For this review, take the finished solid that the model builds, in its own axes (mm). Face numbers are marked on the shaded views. Give positions to 0.01 mm unless a question says otherwise; leave off trailing zeros. Loops run counter-clockwise (first coordinate to the right, second up) from the corner with the lowest first, then second, coordinate; pieces in that order, holes last. Notation, with made-up numbers: (84, 81) - (117, 81) arc R25 ccw to (117, 115) - close; hole circle Ø11 at (74, 39.25). An arc over 180 degrees is marked (long way). Put each result on its own line as item: value.
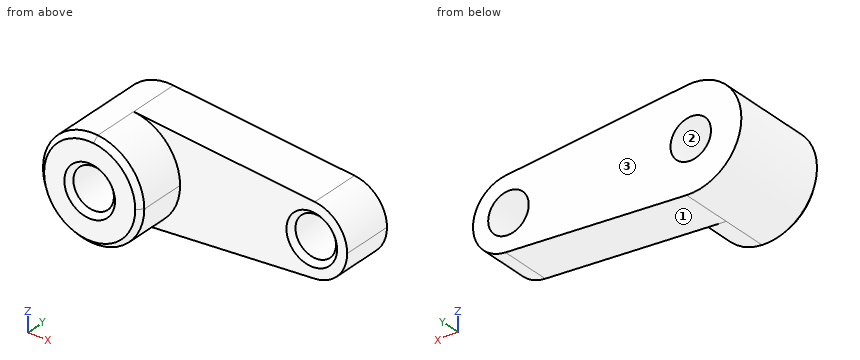
from build123d import *

# Parameters (mm, degrees)
F0_R     = 10
F1_DEPTH = 25
F2_DEPTH = 50
F3_SIZE  = 2.5


with BuildPart() as f1:
    # F0 (on Front) → F1 (new body)
    with BuildSketch(Plane.XZ):
        with BuildLine():
            ThreePointArc((2.083333, 24.913043), (18.399502, 16.92508), (25, 0))
            ThreePointArc((25, 0), (18.399502, -16.92508), (2.083333, -24.913043))
            Line((2.083333, -24.913043), (91.458333, -17.43913))
            ThreePointArc((91.458333, -17.43913), (72.5, 0), (91.458333, 17.43913))
            Line((91.458333, 17.43913), (2.083333, 24.913043))
        make_face()
        with BuildLine():
            ThreePointArc((2.083333, -24.913043), (18.399502, -16.92508), (25, 0))
            ThreePointArc((25, 0), (18.399502, 16.92508), (2.083333, 24.913043))
            ThreePointArc((2.083333, 24.913043), (-25, 0), (2.083333, -24.913043))
        make_face()
        Circle(F0_R, mode=Mode.SUBTRACT)
        with BuildLine():
            ThreePointArc((107.5, 0), (102.879651, 11.847556), (91.458333, 17.43913))
            ThreePointArc((91.458333, 17.43913), (72.5, 0), (91.458333, -17.43913))
            ThreePointArc((91.458333, -17.43913), (102.879651, -11.847556), (107.5, 0))
        make_face()
        with Locations((90, 0)):
            Circle(F0_R, mode=Mode.SUBTRACT)
    extrude(amount=F1_DEPTH)

    # F0 (on Front) → F2 (join)
    with BuildSketch(Plane.XZ):
        with BuildLine():
            ThreePointArc((2.083333, -24.913043), (18.399502, -16.92508), (25, 0))
            ThreePointArc((25, 0), (18.399502, 16.92508), (2.083333, 24.913043))
            ThreePointArc((2.083333, 24.913043), (-25, 0), (2.083333, -24.913043))
        make_face()
        Circle(F0_R, mode=Mode.SUBTRACT)
    extrude(amount=F2_DEPTH)

    # F3
    f3_edges = [f1.edges().sort_by_distance(p)[0] for p in [
        (-2.083333, -50, 24.913043),
        (-10, -50, 0),
        (80, -25, 0),
    ]]
    chamfer(f3_edges, length=F3_SIZE)


solid = f1.part
1) Take a section at A-A on x = 0. State the section outline as (y, z) points, and give its area (3 significant figures).
Geometry check:
outline: (-50, -22.5) - (-47.5, -25) - (0, -25) - (0, -10) - (-47.5, -10) - (-50, -12.5) - close; (-50, 12.5) - (-47.5, 10) - (0, 10) - (0, 25) - (-47.5, 25) - (-50, 22.5) - close
area: 1,490 mm²
2) Wall thickness on line 1 (Z direction, x = 0, y = -12); line 2 (X direction, y = -22, z = -1); line 3 (X direction, y = -23.5, z = 7.5): over which ranges is each line inside the solid? List them lowest first.
Geometry check:
line 1: z = -25 to -10, 10 to 25
line 2: x = -24.98 to -9.95, 9.95 to 80.05, 99.95 to 107.47
line 3: x = -23.85 to -6.61, 6.61 to 81.95, 98.05 to 105.81
3) Take a section at B-B on y = -16. State the section outline as (x, z) points, and give its area (3 significant figures).
Geometry check:
outline: (2.08, -24.91) - (91.46, -17.44) arc R17.5 ccw to (91.46, 17.44) - (2.08, 24.91) arc R25 ccw (long way) to start; hole circle Ø20 at (0, 0); hole circle Ø20 at (90, 0)
area: 4,670 mm²
4) Take a section at D-D on x = 90. State the section outline as (y, z) points.
Geometry check:
outline: (-25, -17.56) - (0, -17.56) - (0, -10) - (-22.5, -10) - (-25, -12.5) - close; (-25, 12.5) - (-22.5, 10) - (0, 10) - (0, 17.56) - (-25, 17.56) - close
5) Take a section at C-C on y = -38. State the section outline as (x, z) points, and give its area (3 significant figures).
Geometry check:
outline: (2.08, -24.91) arc R25 ccw to (25, 0) arc R25 ccw to (2.08, 24.91) arc R25 ccw (long way) to start; hole circle Ø20 at (0, 0)
area: 1,650 mm²
6) Insertion check: pin 1 Ø6 at (x, y) = (82.5, -26) entering from +Z; pin 2 Ø10 at (y, z) = (-35.5, -9) entering from -X; pin 3 Ø5 at (x, y) = (6.5, -37) entering from -Z. Each pin has a flat end and moves straight along its axis. Give the tip position at first contact, or say it passes through.
Geometry check:
pin 1: stops at z = 18.42
pin 2: stops at x = -24.68
pin 3: stops at z = -24.68
7) Draft analysis for pull direction X (two halves, no side actions). For the marked faces 1, 2 and 3, state which applies: pulls with the +X half, pulls with the -X half, needs draft (parallel to the pull), parting line crosses it, or undercut.
Geometry check:
face 1: pulls with the +X half
face 2: undercut
face 3: needs draft
